Autodesk Inventor part; units mm, degrees
ref_plane "YZ Plane" through (0, 0, 0) normal (1, 0, 0) x (0, 1, 0)
ref_plane "XZ Plane" through (0, 0, 0) normal (0, 1, 0) x (-1, 0, 0)
ref_plane "XY Plane" through (0, 0, 0) normal (0, 0, 1) x (1, 0, 0)
sketch "Sketch1" plane through (0, 0, 0) normal (0, 1, 0) x (-1, 0, 0)
  line L0 (7.5, 15) -> (-7.5, 15)
  line L1 (-7.5, 15) -> (-7.5, -15)
  line L2 (-7.5, -15) -> (7.5, -15)
  line L3 (7.5, -15) -> (7.5, 15)
  circle A0 centre (0, 13.65) radius 0.675
  circle A1 centre (0, 9.75) radius 0.675
  circle A2 centre (0, 5.85) radius 0.675
  circle A3 centre (0, 1.95) radius 0.675
  circle A4 centre (0, -1.95) radius 0.675
  circle A5 centre (0, -5.85) radius 0.675
  circle A6 centre (0, -9.75) radius 0.675
  circle A7 centre (0, -13.65) radius 0.675
  point P0 (0, 0)
  point P1 (7.5, 0)
  point P2 (0, 15)
  dimension "d0" = 15
  dimension "d1" = 30
  dimension "d2" = 1.35
  dimension "d3" = 1.35
  dimension "d6" = 3.9
  dimension "d27" = 1.35
extrude "Cuerpo" add sketch "Sketch1" along normal mid plane 10
sketch "Sketch2" plane through (7.5, -5, -15) normal (1, 0, 0) x (0, 0, -1)
  point P0 (-15, 5)
  point P1 (-15, 5)
hole "BCAM3" at (7.5, 0, 0) direction (-1, 0, 0) diameter 3 depth 6 tip angle 118 countersink diameter 6 countersink angle 90
sketch "Sketch3" plane through (-7.5, -5, 15) normal (-1, 0, 0) x (0, 0, 1)
  circle A0 centre (-15, 5) radius 3
hole "M3X0.6" at (-7.5, 0, 0) direction (1, 0, 0) diameter 2.459 end through all
properties part number "Prensa FO"
Can you work these out from the model? Positions are in its coordinate system, mm. A direction names the side the tool comes from. Give positions to 0.01 mm unless a question says otherwise; leave off trailing zeros. Loops run counter-clockwise (first coordinate to the right, second up) from the corner with the lowest first, then second, coordinate; pieces in that order, holes last. Notation, with made-up numbers: (-33, 66.5) - (8, 66.5) arc R30 ccw to (8, 98.5) - close; hole circle Ø7 at (21, -9). An arc over 180 degrees is marked (long way). Return JSON: item names as keys, results as strings.
1. We'd pull the mould along Z, two halves only. Please class faces 3 (the face through (0.09, -0.07, -6.52)), 4 (the face through (0, 0, -15)), 5 (the face through (7.5, 0, 4)): +Z half, -Z half, draft (parallel to the pull), parting line (faces both ways), or undercut.
Output values:
{"face 3": "undercut", "face 4": "-Z half", "face 5": "draft"}
2. For faces 1 (the face through (0, -5, 0)), 2 (the face through (3.72, -0.07, 1.5)), which set-ups out of +Z, -Z, +X, -X, +Y, -Y let a thin tool reach every point of the face, with its end or its side?
Output values:
{"face 1": "+Z, -Z, +X, -X, -Y", "face 2": "+X"}
3. If I drill on line 1 (Z direction, x = 3, y = 0); line 2 (Z direction, x = 3.75, y = -1); line 3 (Y direction, x = 2, z = 0.5), over which ranges is the centre line in solid material (lowest first)?
Output values:
{"line 1": "z = -15 to -1.5, 1.5 to 15", "line 2": "z = -15 to -1.12, 1.12 to 15", "line 3": "y = -5 to -1.41, 1.41 to 5"}
4. I want a section at C-C on y = -4. Give the number of separate pieces and of enclosed holes in the cut face, and give its area (3 significant figures).
Output values:
{"separate pieces": "1", "enclosed holes": "8", "area": "439 mm²"}
5. I want a section at D-D on x = -2. Please give me the cut outline in (y, z), and give its area (3 significant figures).
Output values:
{"outline": "(-5, -15) - (5, -15) - (5, 15) - (-5, 15) - close; hole circle Ø2.46 at (0, 0)", "area": "295 mm²"}
6. I want a section at A-A on z = 5.85. Please give me the cut outline in (x, y) (3 decimals), and give its area (4 significant figures).
Output values:
{"outline": "(-7.5, -5) - (-0.675, -5) - (-0.675, 5) - (-7.5, 5) - close; (0.675, -5) - (7.5, -5) - (7.5, 5) - (0.675, 5) - close", "area": "136.5 mm²"}
7. I want a section at B-B on x = 5. Please give me the cut outline in (y, z), and give its area (3 significant figures).
Output values:
{"outline": "(-5, -15) - (5, -15) - (5, 15) - (-5, 15) - close; hole circle Ø3 at (0, 0)", "area": "293 mm²"}
